The model under review builds one solid part; all positions refer to its coordinate system, in mm. A direction names the side the tool comes from. Coordinates: 2 decimals unless noted, no trailing zeros. Write each loop counter-clockwise with the first axis right and the second up, starting at its lowest first coordinate (ties: lowest second). Pieces come first, ordered by that corner, then holes. Notation, with made-up numbers: (6, 83.5) - (57, 83.5) arc R15 cw to (57, 98.5) - close; hole circle Ø2 at (69.5, -16). An arc over 180 degrees is marked (long way). Put each result on its own line as item: value. Start each with the question number.
Item 1: For pin 1 (1.4 mm diameter, centred on y = -5.5, z = 2, fed in from -X); pin 2 (1.6 mm diameter, centred on y = -2, z = -5, fed in from +X); pin 3 (0.8 mm diameter, centred on x = 1, y = -6.5, fed in from -Z), all flat-tipped, find the tip position at first contact; note any pin that passes through.
Item 2: Consider section A-A on x = -3.6. Give the boundary of the cut face in (y, z).
Item 3: Machinability: for faces 4 (the face through (-2, -2, 0.4)), 5 (the face through (-1, -2, -2.7)), 6 (the face through (-3.493, -1.096, -4.73)), which of the approach directions +Z, -Z, +X, -X, +Y, -Y give a long, thin tool a straight path to every point of the face, cutting with its end or side? Answer none if there is none.
Item 4: Mouldability with a two-part tool opening along Z and no side actions: class faces 1 (the face through (-2, -2, 2.2)), 2 (the face through (1, -7, 0)), 3 (the face through (-1, 0, 0)) as pulls with the +Z half, pulls with the -Z half, needs draft (parallel to the pull), parting line crosses it, or undercut.
Item 5: Consider section C-C on y = -1.65. Give the boundary of the cut face in (x, z), then the cut area to 3 significant figures.
Item 6: To check wall thickness, follow L1, parallel to Z at x = -3.25, y = -1.65; L2, parallel to Z at x = -3.6, y = -3; L3, parallel to Z at x = -2.05, y = -2. State the ranges of each line that lie inside material, in increasing order. Write a range as [from, to].
Item 7: Consider section D-D on x = -2. Give the boundary of the cut face in (y, z), then the cut area to 3 significant figures.
Item 8: Consider section B-B on z = -4.5. Give the boundary of the cut face in (x, y).
```python
from build123d import *

# Parameters (mm, degrees)
SKETCH_1_W          = 2.9
SKETCH_1_H          = 11.5
EXTRUDE_1_DEPTH     = 1.6
SKETCH_2_W          = 0.7
SKETCH_2_H          = 3.3
SKETCH_2_W_2        = 0.4
EXTRUDE_2_DEPTH     = 4
SKETCH_3_W          = 5.6
SKETCH_3_H          = 3.3
EXTRUDE_3_DEPTH     = 3
SKETCH_4_W          = 1
SKETCH_4_H          = 3.3
EXTRUDE_4_DEPTH     = 3
SKETCH_5_R          = 0.6
CUT_EXTRUDE_1_DEPTH = 14.762630563
SKETCH_6_W          = 4.6
SKETCH_6_H          = 3.3
CUT_EXTRUDE_2_DEPTH = 0.3


with BuildPart() as part:
    # 草图1 → 凸台-拉伸1 (new body)
    with BuildSketch(Plane(origin=(0, 0, 0), x_dir=(0, 0, -1), z_dir=(1, 0, 0))):
        with Locations((-1.45, -5.75)):
            Rectangle(SKETCH_1_W, SKETCH_1_H)
    extrude(amount=EXTRUDE_1_DEPTH)

    # 草图2 → 凸台-拉伸2 (add)
    with BuildSketch(Plane.ZY):
        with Locations((2.55, -1.65)):
            Rectangle(SKETCH_2_W, SKETCH_2_H)
        with Locations((0.2, -1.65)):
            Rectangle(SKETCH_2_W_2, SKETCH_2_H)
    extrude(amount=EXTRUDE_2_DEPTH)

    # 草图3 → 凸台-拉伸3 (add)
    with BuildSketch(Plane(origin=(0, 0, 0), x_dir=(-1, 0, 0), z_dir=(0, 0, -1))):
        with Locations((1.2, -1.65)):
            Rectangle(SKETCH_3_W, SKETCH_3_H)
    extrude(amount=EXTRUDE_3_DEPTH)

    # 草图4 → 凸台-拉伸4 (add)
    with BuildSketch(Plane(origin=(0, 0, -3), x_dir=(-1, 0, 0), z_dir=(0, 0, -1))):
        with Locations((3.5, -1.65)):
            Rectangle(SKETCH_4_W, SKETCH_4_H)
    extrude(amount=EXTRUDE_4_DEPTH)

    # 草图5 → 切除-拉伸1 (cut, through all)
    with BuildSketch(Plane(origin=(-3, 0, 0), x_dir=(0, 0, -1), z_dir=(1, 0, 0))):
        with Locations(Location((4.5, -1.65, 0), (0, 0, 90))):
            Circle(SKETCH_5_R)
    extrude(amount=-CUT_EXTRUDE_1_DEPTH, mode=Mode.SUBTRACT)

    # 草图6 → 切除-拉伸2 (cut)
    with BuildSketch(Plane(origin=(0, 0, -3), x_dir=(-1, 0, 0), z_dir=(0, 0, -1))):
        with Locations((0.7, -1.65)):
            Rectangle(SKETCH_6_W, SKETCH_6_H)
    extrude(amount=-CUT_EXTRUDE_2_DEPTH, mode=Mode.SUBTRACT)


solid = part.part
```
Report:
1. pin 1: x = 0
1. pin 2: x = -3
1. pin 3: z = 0
2. outline: (-3.3, -6) - (0, -6) - (0, 0.4) - (-3.3, 0.4) - close; (-3.3, 2.2) - (0, 2.2) - (0, 2.9) - (-3.3, 2.9) - close; hole circle Ø1.2 at (-1.65, -4.5)
3. face 4: -X, +Y, -Y
3. face 5: -Z, +X, +Y, -Y
3. face 6: +X, -X
4. face 1: undercut
4. face 2: pulls with the -Z half
4. face 3: needs draft
5. outline: (-4, -6) - (-3, -6) - (-3, -5.1) - (-4, -5.1) - close; (-4, -3.9) - (-3, -3.9) - (-3, -2.7) - (1.6, -2.7) - (1.6, 2.9) - (-4, 2.9) - (-4, 2.2) - (0, 2.2) - (0, 0.4) - (-4, 0.4) - close
5. area: 26.3 mm²
6. L1: [-6, -5.1], [-3.9, 0.4], [2.2, 2.9]
6. L2: [-6, 0.4], [2.2, 2.9]
6. L3: [-2.7, 0.4], [2.2, 2.9]
7. outline: (-3.3, -2.7) - (0, -2.7) - (0, 0.4) - (-3.3, 0.4) - close; (-3.3, 2.2) - (0, 2.2) - (0, 2.9) - (-3.3, 2.9) - close
7. area: 12.5 mm²
8. outline: (-4, -3.3) - (-3, -3.3) - (-3, -2.25) - (-4, -2.25) - close; (-4, -1.05) - (-3, -1.05) - (-3, 0) - (-4, 0) - close
